from build123d import *

# Parameters (mm, degrees)
BOSS_EXTRUDE1_DEPTH        = 5
BOSS_EXTRUDE1_DEPTH_BACK   = 5
SKETCH1_R                  = 7.5
SKETCH1_R_2                = 2.5
BOSS_EXTRUDE1_2_DEPTH      = 5
BOSS_EXTRUDE1_2_DEPTH_BACK = 5
SKETCH1_R_3                = 25
SKETCH1_R_4                = 20
BOSS_EXTRUDE2_DEPTH        = 1
BOSS_EXTRUDE2_DEPTH_BACK   = 1
SKETCH1_3_R                = 20
SKETCH1_3_R_2              = 7.5


with BuildPart() as part:
    # Sketch1 → Boss-Extrude1 (new, two sides: drawn at the far end of the back side and taken through both)
    with BuildSketch(Plane(origin=(0, 0, 0), x_dir=(1, 0, 0), z_dir=(0, 1, 0)).offset(-BOSS_EXTRUDE1_DEPTH_BACK)):
        with Locations(Location((0, 0, 0), (0, 0, 270))):
            Circle(SKETCH1_R)
        with Locations(Location((0, 0, 0), (0, 0, 270))):
            Circle(SKETCH1_R_2, mode=Mode.SUBTRACT)
    extrude(amount=BOSS_EXTRUDE1_DEPTH + BOSS_EXTRUDE1_DEPTH_BACK)



with BuildPart() as body_2:
    # Sketch1 → Boss-Extrude1 2 (new, two sides: drawn at the far end of the back side and taken through both)
    with BuildSketch(Plane(origin=(0, 0, 0), x_dir=(1, 0, 0), z_dir=(0, 1, 0)).offset(-BOSS_EXTRUDE1_2_DEPTH_BACK)):
        with Locations(Location((0, 0, 0), (0, 0, 270))):
            Circle(SKETCH1_R_3)
        with Locations(Location((0, 0, 0), (0, 0, 270))):
            Circle(SKETCH1_R_4, mode=Mode.SUBTRACT)
    extrude(amount=BOSS_EXTRUDE1_2_DEPTH + BOSS_EXTRUDE1_2_DEPTH_BACK)


with BuildPart() as part_1:
    add(part.part)

    add(body_2.part)  # Boss-Extrude2 merges body 2
    # Sketch1_3 → Boss-Extrude2 (add, two sides: drawn at the far end of the back side and taken through both)
    with BuildSketch(Plane(origin=(0, 0, 0), x_dir=(1, 0, 0), z_dir=(0, 1, 0)).offset(-BOSS_EXTRUDE2_DEPTH_BACK)):
        with Locations(Location((0, 0, 0), (0, 0, 270))):
            Circle(SKETCH1_3_R)
        with Locations(Location((0, 0, 0), (0, 0, 270))):
            Circle(SKETCH1_3_R_2, mode=Mode.SUBTRACT)
    extrude(amount=BOSS_EXTRUDE2_DEPTH + BOSS_EXTRUDE2_DEPTH_BACK)


solid = part_1.part
Read the model definition and answer for the solid it produces. Units are mm, in the model's axes. A direction names the side the tool comes from. Round coordinates to 2 decimals unless told otherwise and drop trailing zeros. Write each loop counter-clockwise with the first axis right and the second up, starting at its lowest first coordinate (ties: lowest second). Pieces come first, ordered by that corner, then holes.
Q1. A tool of negligible diameter and unlimited length cuts with its end or side. For faces 1 (the face through (2, -5, -2)), 2 (the face through (0.33, -3.028, -7.493)), 3 (the face through (0, 1, 9)), from which of +Z, -Z, +X, -X, +Y, -Y can it reach the whole face along a straight path? Write none if from no direction.
Values:
face 1: +Z, -Z, +X, -X, -Y
face 2: -Y
face 3: +Y
Q2. Find section B-B on z = 0. Determine the outline of the cut face in (x, y).
Values:
outline: (-25, -5) - (-20, -5) - (-20, -1) - (-7.5, -1) - (-7.5, -5) - (-2.5, -5) - (-2.5, 5) - (-7.5, 5) - (-7.5, 1) - (-20, 1) - (-20, 5) - (-25, 5) - close; (2.5, -5) - (7.5, -5) - (7.5, -1) - (20, -1) - (20, -5) - (25, -5) - (25, 5) - (20, 5) - (20, 1) - (7.5, 1) - (7.5, 5) - (2.5, 5) - close
Q3. The mould has two halves that part along X. Classify faces 4 (the face through (7.509, -0.07, 23.846)), 5 (the face through (0.33, 2.972, -7.493)), 6 (the face through (17, -5, -11)): released by +X, released by -X, zero draft, split by the parting line, or undercut.
Values:
face 4: split by the parting line
face 5: undercut
face 6: zero draft
Q4. Find section C-C on y = 3. Determine the outline of the cut face in (x, z).
Values:
outline: circle Ø50 at (0, 0); circle Ø15 at (0, 0); hole circle Ø40 at (0, 0); hole circle Ø5 at (0, 0)
Q5. Find section A-A on x = 0. Determine the outline of the cut face in (y, z), and give its area (3 significant figures).
Values:
outline: (-5, -25) - (5, -25) - (5, -20) - (1, -20) - (1, -7.5) - (5, -7.5) - (5, -2.5) - (-5, -2.5) - (-5, -7.5) - (-1, -7.5) - (-1, -20) - (-5, -20) - close; (-5, 2.5) - (5, 2.5) - (5, 7.5) - (1, 7.5) - (1, 20) - (5, 20) - (5, 25) - (-5, 25) - (-5, 20) - (-1, 20) - (-1, 7.5) - (-5, 7.5) - close
area: 250 mm2
Q6. Straight lines are drawn through the part: line 1 (X direction, y = -3.15, z = 0); line 2 (Z direction, x = 2, y = -4.5); line 3 (Z direction, x = -5, y = 3.5). For each, find the intervals that lie inside material, in ascending order.
Values:
line 1: x = -25 to -20, -7.5 to -2.5, 2.5 to 7.5, 20 to 25
line 2: z = -24.92 to -19.9, -7.23 to -1.5, 1.5 to 7.23, 19.9 to 24.92
line 3: z = -24.49 to -19.36, -5.59 to 5.59, 19.36 to 24.49
Q7. Flat-ended cylindrical pins translate along their axes: P1, Ø2, axis at y = 0.5, z = -2, coming from the -X side; P2, Ø3, axis at y = -2, z = -16.5, coming from the -X side; P3, Ø1.5, axis at y = 1.5, z = 0, coming from the +X side. Find the tip coordinate at first contact, or state that the pin passes through.
Values:
P1: stops at x = -24.98
P2: stops at x = -20
P3: stops at x = 25
Q8. Find section D-D on z = 14. Determine the outline of the cut face in (x, y).
Values:
outline: (-20.71, -5) - (-14.28, -5) - (-14.28, -1) - (14.28, -1) - (14.28, -5) - (20.71, -5) - (20.71, 5) - (14.28, 5) - (14.28, 1) - (-14.28, 1) - (-14.28, 5) - (-20.71, 5) - close
